Can you work these out from the model? Positions are in its coordinate system, mm. A direction names the side the tool comes from. Give positions to 0.01 mm unless a question says otherwise; leave off trailing zeros. Order: outer loops, then holes, each group sorted by start corner. A loop starts at its lowest first (then second) coordinate and runs counter-clockwise, first axis right, second up.
Item 1: I'm going to push flat-ended pins straight in: pin 1 Ø1.5 at (x, z) = (58, -89) entering from -Y; pin 2 Ø8 at (y, z) = (182, -77.5) entering from -X; pin 3 Ø8 at (x, z) = (106.5, -128.5) entering from +Y. Where does each tip first touch, or does it pass through?
Item 2: Which directions (+Z, -Z, +X, -X, +Y, -Y) give clear straight access to the entire face, cutting with the end or side of a thin tool? Please do faces 1 (the flat face through (123, 123, -72)), 2 (the flat face through (61, 249, -75)), 3 (the flat face through (61, -4, 4)), 4 (the flat face through (0, 123, -72)), 5 (the flat face through (61, 0, -75)).
Item 3: I want a section at C-C, the plane z = -51.5. Write out the boundary of the cut face in (x, y).
Item 4: If I drill on line 1 along X through (y, z) = (174, -85); line 2 along Y through (x, z) = (81, -26), over which ranges is the centre line in solid material (lowest first)?
Item 5: I want a section at A-A, the plane y = 164. Write out the boundary of the cut face in (x, z), then the cut area to 3 significant figures.
Item 6: I want a section at B-B, the plane x = 15.5. Write out the boundary of the cut face in (y, z).
```python
from build123d import *

# Parameters (mm, degrees)
SKETCH3_W                = 123
SKETCH3_H                = 147
BOSS_EXTRUDE1_DEPTH      = 249
BOSS_EXTRUDE2_DEPTH      = 253
BOSS_EXTRUDE2_DEPTH_BACK = 4
SKETCH4_W                = 131
SKETCH4_H                = 8


with BuildPart() as part:
    # Sketch3 → Boss-Extrude1 (new body)
    with BuildSketch(Plane(origin=(0, 0, 0), x_dir=(1, 0, 0), z_dir=(0, 1, 0))):
        with Locations((61.5, 73.5)):
            Rectangle(SKETCH3_W, SKETCH3_H)
    extrude(amount=BOSS_EXTRUDE1_DEPTH)

    # Sketch4 → Boss-Extrude2 (add, two sides: drawn at the far end of the back side and taken through both)
    with BuildSketch(Plane(origin=(0, 0, 0), x_dir=(1, 0, 0), z_dir=(0, 1, 0)).offset(-BOSS_EXTRUDE2_DEPTH_BACK)):
        with Locations((61.5, -4)):
            Rectangle(SKETCH4_W, SKETCH4_H)
    extrude(amount=BOSS_EXTRUDE2_DEPTH + BOSS_EXTRUDE2_DEPTH_BACK)


solid = part.part
```
Results list:
1. pin 1: stops at y = 0
1. pin 2: stops at x = 0
1. pin 3: stops at y = 249
2. face 1: -Z, +X, +Y, -Y
2. face 2: -Z, +X, -X, +Y
2. face 3: +Z, -Z, +X, -X, -Y
2. face 4: -Z, -X, +Y, -Y
2. face 5: -Z, +X, -X, -Y
3. outline: (0, 0) - (123, 0) - (123, 249) - (0, 249) - close
4. line 1: x = 0 to 123
4. line 2: y = 0 to 249
5. outline: (-4, 0) - (0, 0) - (0, -147) - (123, -147) - (123, 0) - (127, 0) - (127, 8) - (-4, 8) - close
5. area: 19,100 mm2
6. outline: (-4, 0) - (0, 0) - (0, -147) - (249, -147) - (249, 0) - (253, 0) - (253, 8) - (-4, 8) - close
